```python
from build123d import *

# Parameters (mm, degrees)
SKETCH1_W                      = 127.635
SKETCH1_H                      = 127.635
MAIN_PLATE_DEPTH               = 12.7
SKETCH9_R                      = 83.82
BOSS_EXTRUDE1_DEPTH            = 12.7
SKETCH10_R                     = 97.039626961
SKETCH10_R_2                   = 83.82
CUT_EXTRUDE1_DEPTH             = 167.64
SKETCH2_R                      = 3.556
U_BOLT_HOLE_DEPTH              = 12.7
U_BOLT_PATTERN_COUNT           = 2
U_BOLT_PATTERN_PITCH           = 34.925
U_BOLT_PATTERN_COUNT_DIR2      = 2
U_BOLT_PATTERN_PITCH_DIR2      = 89.535
SKETCH3_R                      = 1.778
RAPTOR_BOLT_HOLE_DEPTH         = 12.7
RAPTOR_BOLT_PATTERN_COUNT      = 2
RAPTOR_BOLT_PATTERN_PITCH      = 38.1
RAPTOR_BOLT_PATTERN_COUNT_DIR2 = 2
RAPTOR_BOLT_PATTERN_PITCH_DIR2 = 76.835
SKETCH4_R                      = 12.7
CO2_CYLINDER_HOLE_DEPTH        = 12.7
CO2_PATTERN_COUNT              = 2
CO2_PATTERN_PITCH              = 76.835


with BuildPart() as part:
    # Sketch1 → Main Plate (new body)
    with BuildSketch(Plane(origin=(0, 0, 0), x_dir=(1, 0, 0), z_dir=(0, 1, 0))):
        with Locations((63.8175, 63.8175)):
            Rectangle(SKETCH1_W, SKETCH1_H)
    extrude(amount=MAIN_PLATE_DEPTH)

    # Sketch9 → Boss-Extrude1 (add)
    with BuildSketch(Plane(origin=(0, 12.7, 0), x_dir=(1, 0, 0), z_dir=(0, 1, 0))):
        with Locations((63.8175, 63.8175)):
            Circle(SKETCH9_R)
    extrude(amount=-BOSS_EXTRUDE1_DEPTH)

    # Sketch10 → Cut-Extrude1 (cut)
    with BuildSketch(Plane(origin=(0, 12.7, 0), x_dir=(1, 0, 0), z_dir=(0, 1, 0))):
        with Locations((63.8175, 63.8175)):
            Circle(SKETCH10_R)
        with Locations((63.8175, 63.8175)):
            Circle(SKETCH10_R_2, mode=Mode.SUBTRACT)
    extrude(amount=-CUT_EXTRUDE1_DEPTH, mode=Mode.SUBTRACT)

    # Sketch2 → U-Bolt Hole (cut)
    with BuildSketch(Plane(origin=(0, 12.7, 0), x_dir=(1, 0, 0), z_dir=(0, 1, 0))):
        with Locations((46.355, 108.585)):
            Circle(SKETCH2_R)
    u_bolt_hole = extrude(amount=-U_BOLT_HOLE_DEPTH, mode=Mode.SUBTRACT)

    # U-Bolt Pattern: U-Bolt Hole 2 × 2
    with Locations(*[(i * U_BOLT_PATTERN_PITCH, 0, j * U_BOLT_PATTERN_PITCH_DIR2) for i in range(U_BOLT_PATTERN_COUNT) for j in range(U_BOLT_PATTERN_COUNT_DIR2) if (i, j) != (0, 0)]):
        add(u_bolt_hole, mode=Mode.SUBTRACT)

    # Sketch3 → Raptor Bolt Hole (cut)
    with BuildSketch(Plane(origin=(0, 12.7, 0), x_dir=(1, 0, 0), z_dir=(0, 1, 0))):
        with Locations((25.4, 44.7675)):
            Circle(SKETCH3_R)
    raptor_bolt_hole = extrude(amount=-RAPTOR_BOLT_HOLE_DEPTH, mode=Mode.SUBTRACT)

    # Raptor Bolt Pattern: Raptor Bolt Hole 2 × 2
    with Locations(*[(j * RAPTOR_BOLT_PATTERN_PITCH_DIR2, 0, -i * RAPTOR_BOLT_PATTERN_PITCH) for i in range(RAPTOR_BOLT_PATTERN_COUNT) for j in range(RAPTOR_BOLT_PATTERN_COUNT_DIR2) if (i, j) != (0, 0)]):
        add(raptor_bolt_hole, mode=Mode.SUBTRACT)

    # Sketch4 → Co2 Cylinder Hole (cut)
    with BuildSketch(Plane(origin=(0, 12.7, 0), x_dir=(1, 0, 0), z_dir=(0, 1, 0))):
        with Locations((25.4, 63.8175)):
            Circle(SKETCH4_R)
    co2_cylinder_hole = extrude(amount=-CO2_CYLINDER_HOLE_DEPTH, mode=Mode.SUBTRACT)

    # Co2 Pattern: Co2 Cylinder Hole ×2
    with Locations(*[(i * CO2_PATTERN_PITCH, 0, 0) for i in range(1, CO2_PATTERN_COUNT)]):
        add(co2_cylinder_hole, mode=Mode.SUBTRACT)


solid = part.part
```
Can you work these out from the model? Positions are in its coordinate system, mm. Coordinates: 2 decimals unless noted, no trailing zeros. Loops run counter-clockwise (first coordinate to the right, second up) from the corner with the lowest first, then second, coordinate; pieces in that order, holes last.
Item 1: Suppose I cut it at B-B (x = 81.28). Please give me the cut outline in (y, z), then the cut area to 3 significant figures.
Answers below:
outline: (0, -145.8) - (12.7, -145.8) - (12.7, -112.14) - (0, -112.14) - close; (0, -105.03) - (12.7, -105.03) - (12.7, -22.61) - (0, -22.61) - close; (0, -15.49) - (12.7, -15.49) - (12.7, 18.16) - (0, 18.16) - close
area: 1,900 mm2
Item 2: Please list where these lines run through material, in increasing order: L1, parallel to X at y = 8, z = -19.5; L2, parallel to Z at x = 25.4, y = 5.5; L3, parallel to X at y = 8.75, z = -111.
Answers below:
L1: x = -7.33 to 42.83, 49.88 to 77.75, 84.81 to 134.96
L2: z = -138.32 to -84.65, -81.09 to -76.52, -51.12 to -46.55, -42.99 to 10.68
L3: x = -5.46 to 43.74, 48.97 to 78.67, 83.89 to 133.1
Item 3: I'm going to push flat-ended pins straight in: pin 1 (3 mm diameter, centred on x = 66, y = 6, fed in from +Z); pin 2 (1 mm diameter, centred on x = 36.5, y = 1.5, fed in from +Z); pin 3 (3 mm diameter, centred on x = 0.5, y = 2.5, fed in from +Z). Where does each tip first touch, or does it pass through?
Answers below:
pin 1: stops at z = 20
pin 2: stops at z = 15.6
pin 3: stops at z = -7.21
Item 4: Suppose I cut it at D-D (z = -115). Please give me the cut outline in (x, y), then the cut area to 3 significant figures.
Answers below:
outline: (-2.56, 0) - (130.2, 0) - (130.2, 12.7) - (-2.56, 12.7) - close
area: 1,690 mm2
Item 5: Suppose I cut it at A-A (z = -19.05). Please give me the cut outline in (x, y).
Answers below:
outline: (-7.05, 0) - (42.8, 0) - (42.8, 12.7) - (-7.05, 12.7) - close; (49.91, 0) - (77.72, 0) - (77.72, 12.7) - (49.91, 12.7) - close; (84.84, 0) - (134.68, 0) - (134.68, 12.7) - (84.84, 12.7) - close
Item 6: Suppose I cut it at C-C (y = 3). State how many separate pieces and enclosed holes the cut face has, then the cut area to 3 significant figures.
Answers below:
separate pieces: 1
enclosed holes: 10
area: 20,900 mm2
Item 7: If we mould it in two halves opening along X, with no side actions, what happens to faces 1 (the face through (108.4, 6.4, -134.8)), 2 (the face through (63, 0, -65)), 3 (the face through (114.35, 6.44, -67.63))? For each: released by +X, released by -X, zero draft, split by the parting line, or undercut.
Answers below:
face 1: split by the parting line
face 2: zero draft
face 3: undercut
